The listing builds one solid part. Answer for the finished solid, in the listing's coordinates (mm). Round coordinates to 2 decimals unless told otherwise and drop trailing zeros. Order: outer loops, then holes, each group sorted by start corner. A loop starts at its lowest first (then second) coordinate and runs counter-clockwise, first axis right, second up. Notation, with made-up numbers: M 86.25,37.25 L 139.25,37.25 A9 ccw 139.25,43.25 Z; hole C 82.5,-31.75 d10. An arc over 180 degrees is marked long. Put each result on its own line as item: value. Start each with the question number.
1. The part is cut by section A-A (y = 1.95). Count the separate pieces of the cut face and the enclosed holes in it, then the cut area to 3 significant figures.
2. The part is cut by section B-B (z = -58.5). Give the vertices of the cut face in (x, y), then the cut area to 3 significant figures.
3. Consider line 1 (X direction, y = 1.45, z = 90.5); line 2 (X direction, y = 1.9, z = -5); line 3 (Z direction, x = 16, y = 1.5). Determine where each line is inside the solid, lowest interval first.
4. Each of these flat-tipped pins is pushed along its axis until it touches: pin 1 Ø1.5 at (x, y) = (-66.5, 1.5) entering from +Z; pin 2 Ø0.9 at (y, z) = (1, 72.5) entering from +X; pin 3 Ø3 at (x, z) = (15, 90.5) entering from +Y; pin 4 Ø4.5 at (x, z) = (-70.5, 15) entering from -Y. Where does it stop, or does it pass through?
from build123d import *

# Parameters (mm, degrees)
SKETCH_1_W          = 97
SKETCH_1_H          = 187
EXTRUDE_1_DEPTH     = 3
SKETCH_4_W          = 25
SKETCH_4_H          = 60
EXTRUDE_2_DEPTH     = 3
SKETCH_6_R          = 1.65
CUT_EXTRUDE_5_DEPTH = 3


with BuildPart() as part:
    # 草图1 → 凸台-拉伸1 (new body)
    with BuildSketch(Plane(origin=(0, 0, 0), x_dir=(1, 0, 0), z_dir=(0, 1, 0))):
        Rectangle(SKETCH_1_W, SKETCH_1_H)
    extrude(amount=EXTRUDE_1_DEPTH)

    # 草图4 → 凸台-拉伸2 (add)
    with BuildSketch(Plane(origin=(0, 3, 0), x_dir=(1, 0, 0), z_dir=(0, 1, 0))):
        with Locations((61, 0)):
            Rectangle(SKETCH_4_W, SKETCH_4_H)
    extrude_2 = extrude(amount=-EXTRUDE_2_DEPTH)

    # 镜向1: 凸台-拉伸2 across plane
    add(extrude_2.mirror(Plane(origin=(0, 0, 0), x_dir=(0, 0, 1), z_dir=(1, 0, 0))))

    # 草图6 → 切除-拉伸5 (cut)
    with BuildSketch(Plane(origin=(0, 3, 0), x_dir=(1, 0, 0), z_dir=(0, 1, 0))):
        with Locations(Location((-5, -90.5, 0), (0, 0, 270))):
            Circle(SKETCH_6_R)
        with Locations(Location((15, -90.5, 0), (0, 0, 270))):
            Circle(SKETCH_6_R)
        with Locations(Location((70.5, -15, 0), (0, 0, 270))):
            Circle(SKETCH_6_R)
        with Locations(Location((70.5, 5, 0), (0, 0, 270))):
            Circle(SKETCH_6_R)
        with Locations(Location((15, 90.5, 0), (0, 0, 270))):
            Circle(SKETCH_6_R)
        with Locations(Location((-5, 90.5, 0), (0, 0, 270))):
            Circle(SKETCH_6_R)
        with Locations(Location((-70.5, -15, 0), (0, 0, 270))):
            Circle(SKETCH_6_R)
        with Locations(Location((-70.5, 5, 0), (0, 0, 270))):
            Circle(SKETCH_6_R)
    extrude(amount=-CUT_EXTRUDE_5_DEPTH, mode=Mode.SUBTRACT)


solid = part.part
Resolved:
1. separate pieces: 1
1. enclosed holes: 8
1. area: 21,100 mm2
2. outline: M -48.5,0 L 48.5,0 L 48.5,3 L -48.5,3 Z
2. area: 291 mm2
3. line 1: -48.5 to -6.65, -3.35 to 13.35, 16.65 to 48.5
3. line 2: -73.5 to -72.15, -68.85 to 68.85, 72.15 to 73.5
3. line 3: -93.5 to -91.81, -89.19 to 89.19, 91.81 to 93.5
4. pin 1: z = 30
4. pin 2: x = 48.5
4. pin 3: through
4. pin 4: y = 0
